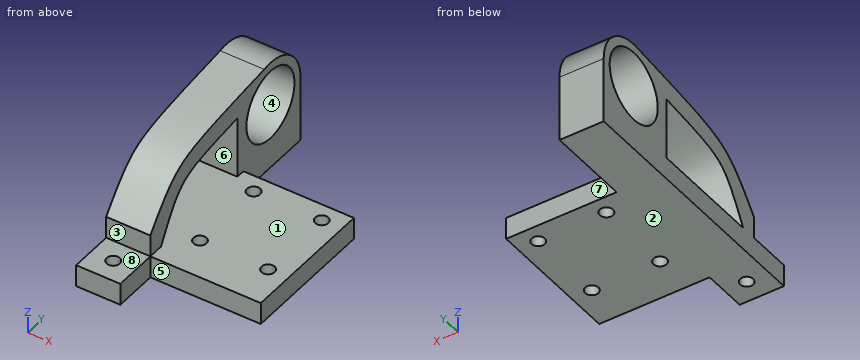
Autodesk Fusion 360 part; units mm, degrees
sketch "Sketch1" plane through (0, 0, 0) normal (0, 0, 1) x (1, 0, 0)
  line L0 (0, 0) -> (20, 0)
  line L1 (20, 0) -> (20, 50)
  line L2 (20, 50) -> (0, 50)
  line L3 (0, 50) -> (0, 0)
  dimension "d1" = 50
extrude "Extrude1" add sketch "Sketch1" along normal blind 30
sketch "Sketch2" plane through (0, 0, 0) normal (0, -1, 0) x (1, 0, 0)
  line L0 (0, 0) -> (20, 0)
  line L1 (20, 0) -> (20, 30)
  line L2 (20, 30) -> (0, 30)
  line L3 (0, 30) -> (0, 0)
  line L4 (0, 30) -> (10, 30)
  line L5 (20, 0) -> (20, 5)
  line L6 (20, 5) -> (10, 5)
  line L7 (10, 5) -> (10, 30)
  dimension "d4" = 5
extrude "Extrude2" cut sketch "Sketch2" against normal blind 70 contours L1 L2 L6 L7
sketch "Sketch3" plane through (0, 0, 0) normal (-1, 0, 0) x (0, -1, 0)
  line L0 (-50, 0) -> (0, 0)
  line L1 (0, 0) -> (0, 30)
  line L2 (0, 30) -> (-50, 30)
  line L3 (-50, 30) -> (-50, 0)
  line L4 (-50, 15) -> (-40, 15)
  line L5 (-40, 15) -> (-40, 30)
  circle A0 centre (-40, 15) radius 8
  dimension "d7" = 16
extrude "Extrude3" cut sketch "Sketch3" against normal blind 15 contours L4 L5 A0 | L4 L5 A0
sketch "Sketch4" plane through (0, 0, 5) normal (0, 0, 1) x (-1, 0, 0)
  line L0 (-20, -50) -> (-10, -50)
  line L1 (-10, -50) -> (-10, 0)
  line L2 (-10, 0) -> (-20, 0)
  line L3 (-20, 0) -> (-20, -50)
  circle A0 centre (-15, -45) radius 0.25
  line L4 (-10, -30) -> (-20, -30)
  circle A1 centre (-15, -27.0301) radius 1.5
  circle A2 centre (-15, -23.4587) radius 1.5
  circle A3 centre (-15, -19.8873) radius 1.5
  circle A4 centre (-15, -16.3158) radius 1.5
  circle A5 centre (-15, -12.7444) radius 1.5
  circle A6 centre (-15, -9.173) radius 1.5
  circle A7 centre (-15, -5.6015) radius 1.5
  circle A8 centre (-15, -2.0301) radius 1.5
  dimension "d11" = 3
  dimension "d14" = 0
  dimension "d15" = 25
extrude "Extrude4" cut sketch "Sketch4" against normal blind 15 contours A1 | A2 | A3 | A4 | A5 | A6 | A7 | A8
sketch "Sketch5" plane through (0, 0, 0) normal (-1, 0, 0) x (0, -1, 0)
  circle A0 centre (-40, 15) radius 8
  line L0 (-50, 0) -> (0, 0)
  line L1 (0, 0) -> (0, 30)
  line L2 (0, 30) -> (-50, 30)
  line L3 (-50, 30) -> (-50, 0)
  circle A1 centre (-40, 15) radius 10
  spline S0 degree 2 poles (-40, 25) (-9.0379, 21.8056) (0, 10) knots 0 0 0 4.447549 4.447549 4.447549 weights 1 3 1
extrude "Extrude5" cut sketch "Sketch5" against normal blind 60 contours L1 L2 L3 A1 S0
sketch "Sketch6" plane through (0, 0, 0) normal (-1, 0, 0) x (0, -1, 0)
  arc A0 (-37.945, 24.7866) -> (-50, 15) centre (-40, 15) ccw
  line L0 (-50, 15) -> (-50, 0)
  line L1 (-50, 0) -> (0, 0)
  line L2 (0, 0) -> (0, 10)
  spline S0 degree 2 poles (0, 10) (-9.0024, 21.7593) (-37.945, 24.7866) knots -4.447549 -4.447549 -4.447549 -0.051947 -0.051947 -0.051947 weights 1 2.97664 1.046174
  circle A1 centre (-40, 15) radius 8
  line L3 (-3, 4) -> (-4, 4)
  line L4 (-4, 4) -> (-29, 4)
  line L5 (-29, 4) -> (-29, 19)
  spline S1 degree 2 poles (-29, 19) (-10, 17) (-3, 4) knots 0 0 0 3.222354 3.222354 3.222354 weights 1 3 1
  line L6 (-3.5416, 5) -> (-29, 5)
extrude "Extrude6" cut sketch "Sketch6" against normal blind 16 contours L5 S1 L6
sketch "Sketch7" plane through (0, 0, 5) normal (0, 0, 1) x (-1, 0, 0)
  circle A0 centre (-15, -9.173) radius 1.5
  circle A1 centre (-15, -5.6015) radius 1.5
  circle A2 centre (-15, -12.7444) radius 1.5
  circle A3 centre (-15, -16.3158) radius 1.5
  line L0 (-10, -3.5416) -> (-10, 0)
  line L1 (-10, 0) -> (-20, 0)
  line L2 (-20, 0) -> (-20, -50)
  line L3 (-20, -50) -> (-10, -50)
  line L4 (-10, -50) -> (-10, -29)
  line L5 (-10, -29) -> (0, -29)
  line L6 (0, -29) -> (0, -3.5416)
  line L7 (0, -3.5416) -> (-10, -3.5416)
  circle A4 centre (-15, -19.8873) radius 1.5
  circle A5 centre (-15, -27.0301) radius 1.5
  circle A6 centre (-15, -23.4587) radius 1.5
  circle A7 centre (-15, -2.0301) radius 1.5
  line L8 (-10, -50) -> (-10, -31)
  line L9 (-20, -31) -> (-10, -31)
  line L10 (-20, -31) -> (-20, -50)
  line L11 (-10, -50) -> (-20, -50)
extrude "Extrude7" cut sketch "Sketch7" against normal blind 15 contours L2 L3 L4 L8 L9 L10 L11
sketch "Sketch8" plane through (0, 0, 0) normal (0, 0, -1) x (1, 0, 0)
  line L0 (10, -31) -> (20, -31)
  line L1 (20, -31) -> (20, 0)
  line L2 (20, 0) -> (0, 0)
  line L3 (0, 0) -> (0, -50)
  line L4 (0, -50) -> (10, -50)
  line L5 (10, -50) -> (10, -31)
  circle A0 centre (15, -19.8873) radius 1.5
  circle A1 centre (15, -5.6015) radius 1.5
  circle A2 centre (15, -9.173) radius 1.5
  circle A3 centre (15, -23.4587) radius 1.5
  circle A4 centre (15, -16.3158) radius 1.5
  circle A5 centre (15, -2.0301) radius 1.5
  circle A6 centre (15, -12.7444) radius 1.5
  circle A7 centre (15, -27.0301) radius 1.5
  circle A8 centre (15, -5.6015) radius 1.5
  circle A9 centre (15, -2.0301) radius 1.5
  circle A10 centre (15, -12.7444) radius 1.5
  circle A11 centre (15, -16.3158) radius 1.5
  circle A12 centre (15, -19.8873) radius 1.5
  circle A13 centre (15, -23.4587) radius 1.5
extrude "Extrude8" add sketch "Sketch8" against normal blind 5 contours A0 A12 | A1 A8 | A3 A13 | A4 A11 | A5 A9 | A6 A10
sketch "Sketch9" plane through (20, 0, 0) normal (1, 0, 0) x (0, 1, 0)
  line L0 (31, 0) -> (31, 5)
  line L1 (31, 5) -> (0, 5)
  line L2 (0, 5) -> (0, 0)
  line L3 (0, 0) -> (31, 0)
extrude "Extrude9" add sketch "Sketch9" along normal blind 15
sketch "Sketch10" plane through (0, 0, 5) normal (0, 0, 1) x (-1, 0, 0)
  line L0 (-35, -31) -> (-10, -31)
  line L1 (-10, -31) -> (-10, -29)
  line L2 (-10, -29) -> (0, -29)
  line L3 (0, -29) -> (0, -3.5416)
  line L4 (0, -3.5416) -> (-10, -3.5416)
  line L5 (-10, -3.5416) -> (-10, 0)
  line L6 (-10, 0) -> (-35, 0)
  line L7 (-35, 0) -> (-35, -31)
  circle A0 centre (-15, -9.173) radius 1.5
  circle A1 centre (-15, -27.0301) radius 1.5
  circle A2 centre (-30.4309, -27.0301) radius 1.5
  circle A3 centre (-30.4309, -9.173) radius 1.5
  dimension "d30" = 3
  dimension "d31" = 3
extrude "Extrude10" cut sketch "Sketch10" against normal blind 40 contours A2 | A3
sketch "Sketch11" plane through (0, 0, 0) normal (0, -1, 0) x (1, 0, 0)
  line L0 (10, 10) -> (0, 10)
  line L1 (0, 10) -> (0, 0)
  line L2 (0, 0) -> (35, 0)
  line L3 (35, 0) -> (35, 5)
  line L4 (35, 5) -> (10, 5)
  line L5 (10, 5) -> (10, 10)
  line L6 (10, 5) -> (0, 5)
  line L7 (0, 0) -> (0, 5)
  line L8 (10, 5) -> (10, 0)
  line L9 (0, 0) -> (10, 0)
extrude "Extrude11" add sketch "Sketch11" along normal blind 10 contours L1 L2 L6 L7 L8 L9
sketch "Sketch12" plane through (0, 0, 5) normal (0, 0, 1) x (-1, 0, 0)
  line L0 (-10, 0) -> (0, 0)
  line L1 (0, 0) -> (0, 10)
  line L2 (0, 10) -> (-10, 10)
  line L3 (-10, 10) -> (-10, 0)
  circle A0 centre (-5, 5) radius 1.5
  dimension "d36" = 3
extrude "Extrude12" cut sketch "Sketch12" against normal blind 15 contours A0
Geometry check sheet. Reference: the model listing, model coordinates, mm. Face numbers are marked on the shaded views. A direction names the side the tool comes from. Coordinates: 2 decimals unless noted, no trailing zeros. Write each loop counter-clockwise with the first axis right and the second up, starting at its lowest first coordinate (ties: lowest second). Pieces come first, ordered by that corner, then holes. Notation, with made-up numbers: (86.5, -0.5) -> (100.5, -0.5) arc R33 cw to (100.5, 32.5) -> close; hole circle Ø4 at (-2, 18.5). An arc over 180 degrees is marked (long way). One line per question, with ' | ' between items.
1. Set-up check for the marked faces 5, 6, 7 and 8: record each of +Z, -Z, +X, -X, +Y, -Y from which the full face is reachable in a straight line by a thin tool's end or side.
Answers:
face 5: +Z, -Z, +X, -Y | face 6: +X, -X | face 7: +Z, -Z, +X, +Y | face 8: +Z, +X, -X, -Y
2. Depth check by flat-ended pin: pin 1 Ø2.5 at (y, z) = (-5.5, 3.5) entering from +X; pin 2 Ø4 at (x, y) = (5, -5) entering from -Z; pin 3 Ø2.5 at (x, z) = (18.5, 2) entering from -Y; pin 4 Ø1.5 at (x, z) = (17.5, 2) entering from +Y. Enter the tip coordinate at first touch or a pass-through.
Answers:
pin 1: stops at x = 10 | pin 2: stops at z = 0 | pin 3: stops at y = 0 | pin 4: stops at y = 31
3. Draft check along Y on the marked faces 1, 2, 3 and 4. Enter one of: +Y half, -Y half, draft (parallel to the pull), parting line (faces both ways), or undercut.
Answers:
face 1: undercut | face 2: draft | face 3: -Y half | face 4: undercut
4. Cross-section at A-A on x = 15. Record the cut outline in (y, z), and give its area (3 significant figures).
Answers:
outline: (0, 0) -> (7.67, 0) -> (7.67, 5) -> (0, 5) -> close; (10.67, 0) -> (25.53, 0) -> (25.53, 5) -> (10.67, 5) -> close; (28.53, 0) -> (31, 0) -> (31, 5) -> (28.53, 5) -> close | area: 125 mm²
5. Cross-section at B-B on y = -5. Record the cut outline in (x, z), and give its area (3 significant figures).
Answers:
outline: (0, 0) -> (3.5, 0) -> (3.5, 5) -> (0, 5) -> close; (6.5, 0) -> (10, 0) -> (10, 5) -> (6.5, 5) -> close | area: 35.0 mm²
6. Cross-section at C-C on z = 2.75. Record the cut outline in (x, y).
Answers:
outline: (0, -10) -> (10, -10) -> (10, 0) -> (35, 0) -> (35, 31) -> (10, 31) -> (10, 50) -> (0, 50) -> close; hole circle Ø3 at (5, -5); hole circle Ø3 at (15, 9.17); hole circle Ø3 at (15, 27.03); hole circle Ø3 at (30.43, 9.17); hole circle Ø3 at (30.43, 27.03)
7. Thickness scan on probe 1 along Y at (x, z) = (15, 2.45); probe 2 along X at (y, z) = (10.5, 3.5); probe 3 along Y at (x, z) = (7.75, 15). Record the ranges inside material, lowest first. Write a range as from..to.
Answers:
probe 1: y = 0..7.67, 10.67..25.53, 28.53..31 | probe 2: x = 0..14.3, 15.7..29.73, 31.13..35 | probe 3: y = 4.06..10.55, 29..32, 48..50
8. Cross-section at D-D on x = 5. State how many separate pieces and enclosed holes the cut face has, and give its area (3 significant figures).
Answers:
separate pieces: 2 | enclosed holes: 2 | area: 639 mm²
